Geometry: final body of the model. Coordinates: model frame, mm. A direction names the side the tool comes from. Give positions to 0.01 mm unless a question says otherwise; leave off trailing zeros. Loops run counter-clockwise (first coordinate to the right, second up) from the corner with the lowest first, then second, coordinate; pieces in that order, holes last. Notation, with made-up numbers: M -17,-36.5 L 0,-36.5 A13 cw 0,-23.5 Z; hole C 33.25,-6 d11. An arc over 180 degrees is marked long. Put each result on its own line as item: value.
```python
from build123d import *

# Parameters (mm, degrees)
SKETCH_W        = 26
SKETCH_H        = 66
PAD_DEPTH       = 12
SKETCH001_R     = 4.2
POCKET_DEPTH    = 26.001
POCKET001_DEPTH = 4.5
SKETCH003_R     = 3.2
POCKET002_DEPTH = 12.001
SKETCH004_R     = 4.2
POCKET003_DEPTH = 7
POCKET004_DEPTH = 5.5
POCKET005_DEPTH = 6


with BuildPart() as part:
    # Sketch → Pad (new body)
    with BuildSketch(Plane.XY):
        with Locations((-13, 0)):
            Rectangle(SKETCH_W, SKETCH_H)
    extrude(amount=PAD_DEPTH)

    # Sketch001 (on Face4 of Pad) → Pocket (cut, through all)
    with BuildSketch(Plane(origin=(-26, 0, 0), x_dir=(0, -1, 0), z_dir=(-1, 0, 0))):
        with Locations((-28, 0)):
            Circle(SKETCH001_R)
        with Locations((28, 0)):
            Circle(SKETCH001_R)
    extrude(amount=-POCKET_DEPTH, mode=Mode.SUBTRACT)

    # Sketch002 (on Face8 of Pocket) → Pocket001 (cut)
    with BuildSketch(Plane(origin=(0, 0, 0), x_dir=(1, 0, 0), z_dir=(0, 0, -1))):
        with BuildLine():
            ThreePointArc((-11, -9), (-2, 0), (-11, 9))
            Line((-11, 9), (-26, 9))
            Line((-26, 9), (-26, -9))
            Line((-26, -9), (-11, -9))
        make_face()
    extrude(amount=-POCKET001_DEPTH, mode=Mode.SUBTRACT)

    # Sketch003 (on Face8 of Pocket001) → Pocket002 (cut, through all)
    with BuildSketch(Plane(origin=(0, 0, 0), x_dir=(1, 0, 0), z_dir=(0, 0, -1))):
        with Locations((-11, 0)):
            Circle(SKETCH003_R)
        with Locations((-20, 15)):
            Circle(SKETCH003_R)
        with Locations((-20, -15)):
            Circle(SKETCH003_R)
    extrude(amount=-POCKET002_DEPTH, mode=Mode.SUBTRACT)

    # Sketch004 (on Face3 of Pocket002) → Pocket003 (cut)
    with BuildSketch(Plane.YZ):
        with Locations((-15, 0)):
            Circle(SKETCH004_R)
        with Locations((15, 0)):
            Circle(SKETCH004_R)
    extrude(amount=-POCKET003_DEPTH, mode=Mode.SUBTRACT)

    # Sketch005 (on Face20 of Pocket003) → Pocket004 (cut)
    with BuildSketch(Plane.YZ.offset(-7)):
        Polygon((-9.8, -3.002221), (-9.8, 3.002221), (-15, 6.004443), (-20.2, 3.002221), (-20.2, -3.002221), (-15, -6.004443), align=None)
        Polygon((15, -6.004443), (20.2, -3.002221), (20.2, 3.002221), (15, 6.004443), (9.8, 3.002221), (9.8, -3.002221), align=None)
    extrude(amount=-POCKET004_DEPTH, mode=Mode.SUBTRACT)

    # Sketch006 (on Face5 of Pocket004) → Pocket005 (cut)
    with BuildSketch(Plane.XY.offset(12)):
        Polygon((-14.8, 11.997779), (-14.8, 18.002221), (-20, 21.004443), (-25.2, 18.002221), (-25.2, 11.997779), (-20, 8.995557), align=None)
        Polygon((-14.8, -18.002221), (-14.8, -11.997779), (-20, -8.995557), (-25.2, -11.997779), (-25.2, -18.002221), (-20, -21.004443), align=None)
        Polygon((-5.8, -3.002221), (-5.8, 3.002221), (-11, 6.004443), (-16.2, 3.002221), (-16.2, -3.002221), (-11, -6.004443), align=None)
    extrude(amount=-POCKET005_DEPTH, mode=Mode.SUBTRACT)


solid = part.part
```
Item 1: Mould query, pull axis X, two halves, no side actions, for faces 1 (the flat face through (-10, 9.8, 2)), 2 (the flat face through (-19, 9, 2)), 3 (the flat face through (-7, -15.8, 4.4)). Classes: pulls with the +X half, pulls with the -X half, needs draft (parallel to the pull), parting line crosses it, or undercut.
Output values:
face 1: undercut
face 2: needs draft
face 3: undercut
Item 2: Line query: probe 1 along Y at (x, z) = (-20, 4.65); probe 2 along Y at (x, z) = (-20, 1.4); probe 3 along X at (y, z) = (15, 4.5). Output: solid intervals per line, ascending. Write a range as [from, to].
Output values:
probe 1: [-33, -18.2], [-11.8, 11.8], [18.2, 33]
probe 2: [-33, -31.96], [-24.04, -18.2], [-11.8, -9], [9, 11.8], [18.2, 24.04], [31.96, 33]
probe 3: [-26, -23.2], [-16.8, -12.5], [-7, 0]
Item 3: Section B-B on z = 2.25. Count the separate pieces of the cut face and the enclosed holes in it, then the cut area to 3 significant figures.
Output values:
separate pieces: 3
enclosed holes: 2
area: 672 mm²
Item 4: Set-up query: faces 4 (the flat face through (-13, 33, 6)), 5 (the flat face through (-18, -9, 2)), 6 (the flat face through (-9.71, 17.64, 4.48)), 7 (the cylindrical face through (-14.2, -0.1, 5.2)), 8 (the flat face through (-22.64, -19.48, 9.04)). Return all of +Z, -Z, +X, -X, +Y, -Y with unobstructed straight access to the full face (end or side cutting, diameter ignored); none if empty.
Output values:
face 4: +Z, -Z, +X, -X, +Y
face 5: -Z, -X
face 6: -Z
face 7: +Z, -Z
face 8: +Z
Item 5: Section A-A on y = 0. Output: boundary loops of the cut face in (x, z), then the cut area to 3 significant figures.
Output values:
outline: M -26,4.5 L -14.2,4.5 L -14.2,6 L -16.2,6 L -16.2,12 L -26,12 Z; M -7.8,4.5 L -2,4.5 L -2,0 L 0,0 L 0,12 L -5.8,12 L -5.8,6 L -7.8,6 Z
area: 132 mm²
Item 6: Section C-C on x = -22. Output: boundary loops of the cut face in (y, z), then the cut area to 3 significant figures.
Output values:
outline: M -33,0 L -32.2,0 A4.2 cw -23.8,0 L -17.5,0 L -17.5,6 L -19.85,6 L -19.85,12 L -33,12 Z; M -12.5,0 L -9,0 L -9,4.5 L 9,4.5 L 9,0 L 12.5,0 L 12.5,6 L 10.15,6 L 10.15,12 L -10.15,12 L -10.15,6 L -12.5,6 Z; M 17.5,0 L 23.8,0 A4.2 cw 32.2,0 L 33,0 L 33,12 L 19.85,12 L 19.85,6 L 17.5,6 Z
area: 479 mm²
Item 7: Pin query (flat end, axial travel): pin 1 Ø5.5 at (x, y) = (-15.5, 0) entering from -Z; pin 2 Ø3 at (x, y) = (-21, 15) entering from +Z; pin 3 Ø1.8 at (y, z) = (15.5, 3) entering from +X. Return the tip coordinate at first contact, or that it passes through.
Output values:
pin 1: z = 4.5
pin 2: through
pin 3: x = -12.5
